Answer from the drawing. Dimensions are ordinates in mm from the lowest x, y and z of the part. A direction names the side the tool comes from. Round coordinates to 2 decimals unless told otherwise and drop trailing zeros. Loops run counter-clockwise (first coordinate to the right, second up) from the corner with the lowest first, then second, coordinate; pieces in that order, holes last. Notation, with made-up numbers: (-18, 43) - (7, 43) arc R24 ccw to (7, 77) - close; hole circle Ø11 at (-32.5, -37.75). An arc over 180 degrees is marked (long way). Write item = value, one per line. Start each with the question number.
1) Section B-B, the plane x = 48.5 is taken. Determine the outline of the cut face in (y, z), and give its area (3 significant figures).
2) A tool of negligible diameter and unlimited length cuts with its end or side. For the marked faces 1, 2 and 3, from which of +Z, -Z, +X, -X, +Y, -Y can it reach the whole face along a straight path? Write none if from no direction.
3) For a pull along Y with two mould halves and no side action, classify the marked faces 4, 5 and 6 as released by +Y, released by -Y, zero draft, split by the parting line, or undercut.
4) Given pin 1 Ø8 at (y, z) = (8, 16) entering from +X; pin 2 Ø9 at (x, y) = (6.5, 9) entering from +Z; pin 3 Ø1.5 at (x, y) = (28, 10.5) entering from -Z, each flat-ended and moving along its own axis, determine where each tip first touches the part or whether it passes through.
5) Section D-D, the plane z = 24.5 is taken. Determine the outline of the cut face in (x, y), and give its area (3 significant figures).
6) Straight lines are drawn through the part: line 1 along X through (y, z) = (9, 4); line 2 along Y through (x, z) = (35.75, 24.5); line 3 along X through (y, z) = (10, 30). For each, find the intervals that lie inside material, in ascending order.
7) Section A-A, the plane z = 6 is taken. Determine the outline of the cut face in (x, y), and give its area (3 significant figures).
8) Section C-C, the plane y = 14.25 is taken. Determine the outline of the cut face in (x, z), and give its area (3 significant figures).
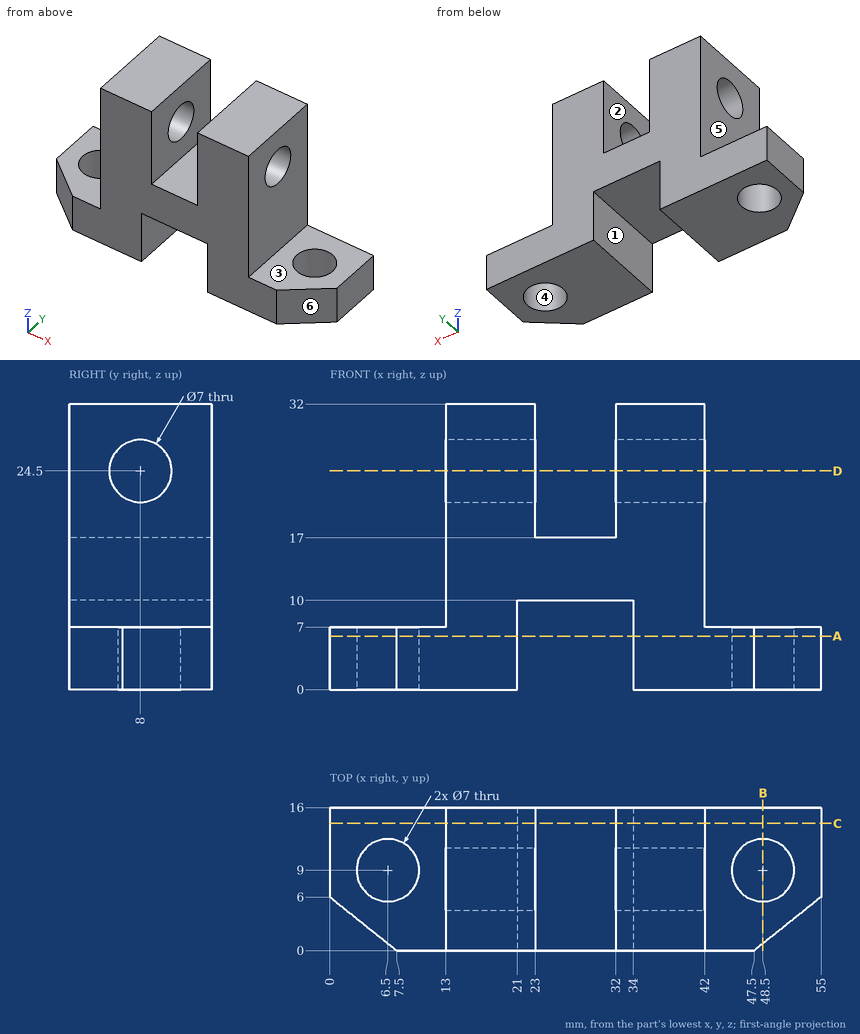
Geometry check:
q1.outline = (0.8, 0) - (5.5, 0) - (5.5, 7) - (0.8, 7) - close; (12.5, 0) - (16, 0) - (16, 7) - (12.5, 7) - close
q1.area = 57.4 mm2
q2.face_1 = -Z, +Y, -Y
q2.face_2 = +Z, +Y, -Y
q2.face_3 = +Z, +X, +Y, -Y
q3.face_4 = undercut
q3.face_5 = zero draft
q3.face_6 = released by -Y
q4.pin_1 = 42
q4.pin_2 = 7
q4.pin_3 = 10
q5.outline = (13, 0) - (23, 0) - (23, 4.5) - (13, 4.5) - close; (13, 11.5) - (23, 11.5) - (23, 16) - (13, 16) - close; (32, 0) - (42, 0) - (42, 4.5) - (32, 4.5) - close; (32, 11.5) - (42, 11.5) - (42, 16) - (32, 16) - close
q5.area = 180 mm2
q6.line_1 = 0 to 3, 10 to 21, 34 to 45, 52 to 55
q6.line_2 = 0 to 4.5, 11.5 to 16
q6.line_3 = 13 to 23, 32 to 42
q7.outline = (0, 6) - (7.5, 0) - (21, 0) - (21, 16) - (0, 16) - close; (34, 0) - (47.5, 0) - (55, 6) - (55, 16) - (34, 16) - close; hole circle Ø7 at (6.5, 9); hole circle Ø7 at (48.5, 9)
q7.area = 550 mm2
q8.outline = (0, 0) - (21, 0) - (21, 10) - (34, 10) - (34, 0) - (55, 0) - (55, 7) - (42, 7) - (42, 32) - (32, 32) - (32, 17) - (23, 17) - (23, 32) - (13, 32) - (13, 7) - (0, 7) - close
q8.area = 845 mm2
